from build123d import *

# Parameters (mm, degrees)
SKIZZE1_R                       = 23.4
SKIZZE1_R_2                     = 1
LINEAR_AUSTRAGEN1_DEPTH         = 2.2
SKIZZE3_R                       = 1.75
SCHNITT_LINEAR_AUSTRAGEN3_DEPTH = 34.165644875


with BuildPart() as part:
    # Skizze1 → Linear austragen1 (new body)
    with BuildSketch(Plane.XY):
        Circle(SKIZZE1_R)
        with Locations((6.643865379, 20.4477151)):
            Circle(SKIZZE1_R_2, mode=Mode.SUBTRACT)
        with Locations((17.393865379, 12.637382924)):
            Circle(SKIZZE1_R_2, mode=Mode.SUBTRACT)
        with Locations((17.393865379, -12.637382924)):
            Circle(SKIZZE1_R_2, mode=Mode.SUBTRACT)
        with Locations((-6.643865379, 20.4477151)):
            Circle(SKIZZE1_R_2, mode=Mode.SUBTRACT)
        with Locations((6.643865379, -20.4477151)):
            Circle(SKIZZE1_R_2, mode=Mode.SUBTRACT)
        with Locations((-6.643865379, -20.4477151)):
            Circle(SKIZZE1_R_2, mode=Mode.SUBTRACT)
        with Locations((-17.393865379, -12.637382924)):
            Circle(SKIZZE1_R_2, mode=Mode.SUBTRACT)
        with Locations((-17.393865379, 12.637382924)):
            Circle(SKIZZE1_R_2, mode=Mode.SUBTRACT)
        with BuildLine():
            ThreePointArc((14.720859381, 11.20474449), (0, 18.5), (-14.720859381, 11.20474449))
            ThreePointArc((-14.720859381, 11.20474449), (-14.883940446, 9.033399462), (-12.967323579, 8))
            ThreePointArc((-12.967323579, 8), (0, 8.526339105), (12.967323579, 8))
            ThreePointArc((12.967323579, 8), (14.883940446, 9.033399462), (14.720859381, 11.20474449))
        make_face(mode=Mode.SUBTRACT)
        with BuildLine():
            ThreePointArc((-14.720859381, -11.20474449), (0, -18.5), (14.720859381, -11.20474449))
            ThreePointArc((14.720859381, -11.20474449), (14.883940446, -9.033399462), (12.967323579, -8))
            ThreePointArc((12.967323579, -8), (0, -8.526339105), (-12.967323579, -8))
            ThreePointArc((-12.967323579, -8), (-14.883940446, -9.033399462), (-14.720859381, -11.20474449))
        make_face(mode=Mode.SUBTRACT)
    extrude(amount=LINEAR_AUSTRAGEN1_DEPTH)

    # Skizze3 → Schnitt-Linear austragen3 (cut, through all)
    with BuildSketch(Plane.XY.offset(2.2)):
        with Locations((12.5, 0)):
            Circle(SKIZZE3_R)
        with Locations(Location((-12.5, 0, 0), (0, 0, 180))):
            Circle(SKIZZE3_R)
        with BuildLine():
            Line((-7.295576741, 5.75), (7.295576741, 5.75))
            ThreePointArc((7.295576741, 5.75), (9.59371007, 4.678362829), (10.25, 2.229055467))
            Line((10.25, 2.229055467), (9.280201606, -3.270944533))
            ThreePointArc((9.280201606, -3.270944533), (8.254141176, -5.048133329), (6.325778347, -5.75))
            Line((6.325778347, -5.75), (-6.325778347, -5.75))
            ThreePointArc((-6.325778347, -5.75), (-8.254141176, -5.048133329), (-9.280201606, -3.270944533))
            Line((-9.280201606, -3.270944533), (-10.25, 2.229055467))
            ThreePointArc((-10.25, 2.229055467), (-9.59371007, 4.678362829), (-7.295576741, 5.75))
        make_face()
    extrude(amount=-SCHNITT_LINEAR_AUSTRAGEN3_DEPTH, mode=Mode.SUBTRACT)


solid = part.part
Can you work these out from the model? Positions are in its coordinate system, mm. Give positions to 0.01 mm unless a question says otherwise; leave off trailing zeros. Order: outer loops, then holes, each group sorted by start corner. A loop starts at its lowest first (then second) coordinate and runs counter-clockwise, first axis right, second up. Notation, with made-up numbers: M -36.75,45 L -19.75,45 A30 ccw -19.75,76 Z; hole C 17.25,-16.75 d9. An arc over 180 degrees is marked long. Use a Markdown table: item, result. Add a question column.
Item 1: If I drill on L1, parallel to X at y = 12.5, z = 0.3; L2, parallel to Y at x = 17, z = 0.45; L3, parallel to Y at x = 12.5, z = 2, over which ranges is the centre line in solid material (lowest first)? Write a range as [from, to].
Item 2: Will these pins go through, and if not, where does the flat tip stop? pin 1 (2.5 mm diameter, centred on x = 17.39, y = 12.64, fed in from -Z); pin 2 (1.1 mm diameter, centred on x = 1.5, z = 0.5, fed in from +Y); pin 3 (1.1 mm diameter, centred on x = 2, z = 1, fed in from -Y); pin 4 (1.6 mm diameter, centred on x = 17.39, y = -12.64, fed in from -Z).
Item 3: Suppose I cut it at C-C (y = -17). List the corners of the cut face in (x, z) for me.
Item 4: Suppose I cut it at B-B (z = 0.7). Count the separate pieces of the cut face and the enclosed holes in it, then the cut area to 3 significant figures.
Item 5: Suppose I cut it at D-D (y = -7). List the corners of the cut face in (x, z) for me.
Item 6: Suppose I cut it at A-A (x = 0). List the corners of the cut face in (y, z) for me.
Answer sheet:
| question | item | result |
|---|---|---|
| 1 | L1 | x = [-19.78, -18.38], [-16.4, -13.64], [13.64, 16.4], [18.38, 19.78] |
| 1 | L2 | y = [-16.08, -13.56], [-11.72, 11.72], [13.56, 16.08] |
| 1 | L3 | y = [-19.78, -13.64], [-8.04, -1.75], [1.75, 8.04], [13.64, 19.78] |
| 2 | pin 1 | stops at z = 0 |
| 2 | pin 2 | stops at y = 23.38 |
| 2 | pin 3 | stops at y = -23.36 |
| 2 | pin 4 | passes through |
| 3 | outline | M -16.08,0 L -7.3,0 L -7.3,2.2 L -16.08,2.2 Z; M 7.3,0 L 16.08,0 L 16.08,2.2 L 7.3,2.2 Z |
| 4 | separate pieces | 1 |
| 4 | enclosed holes | 13 |
| 4 | area | 986 mm² |
| 5 | outline | M -22.33,0 L 22.33,0 L 22.33,2.2 L -22.33,2.2 Z |
| 6 | outline | M -23.4,0 L -18.5,0 L -18.5,2.2 L -23.4,2.2 Z; M -8.53,0 L -5.75,0 L -5.75,2.2 L -8.53,2.2 Z; M 5.75,0 L 8.53,0 L 8.53,2.2 L 5.75,2.2 Z; M 18.5,0 L 23.4,0 L 23.4,2.2 L 18.5,2.2 Z |
